Part print with two shaded views. Sizes in mm from the minimum x, y, z corner. Round coordinates to 2 decimals unless told otherwise and drop trailing zeros. Order: outer loops, then holes, each group sorted by start corner. A loop starts at its lowest first (then second) coordinate and runs counter-clockwise, first axis right, second up. Notation, with made-up numbers: (-26.5, 39) - (17.5, 39) arc R26 ccw to (17.5, 64) - close; hole circle Ø5 at (-14.75, -27). An arc over 180 degrees is marked (long way). Use one line per item in the form item = value.
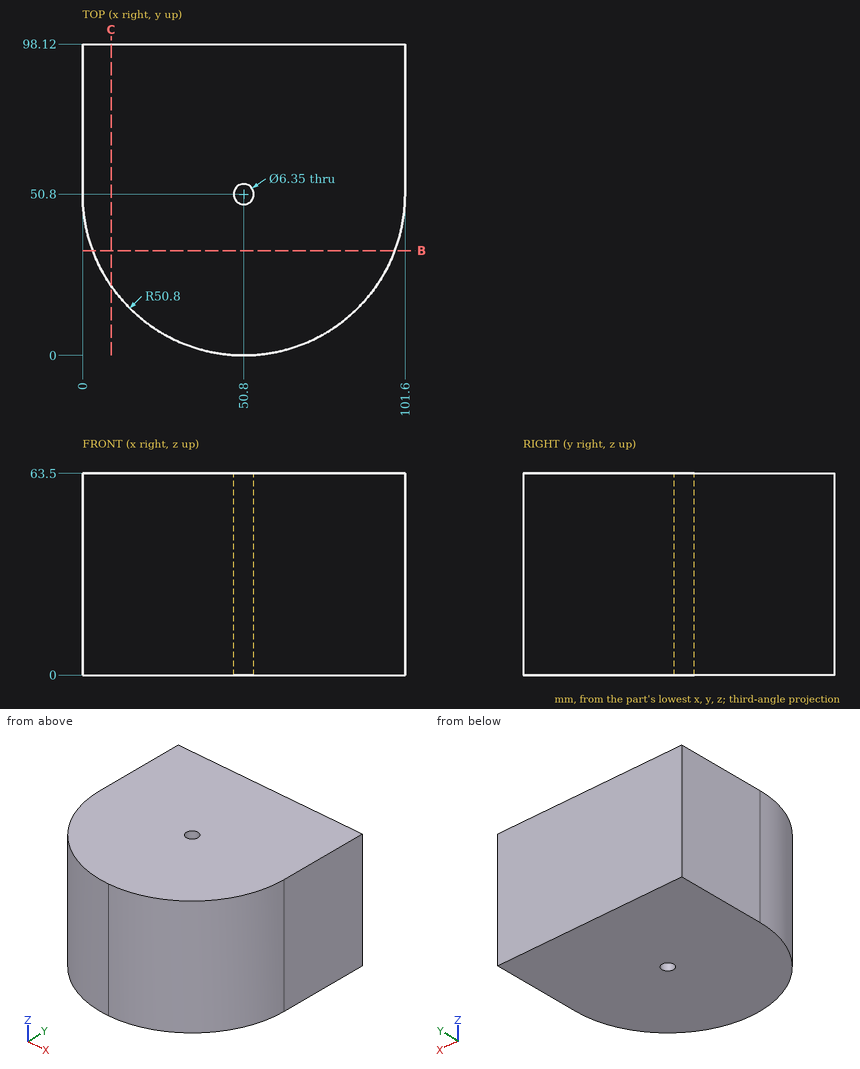
(1) Pin check, flat tips, straight feed: pin 1 (6 mm diameter, centred on x = 71, z = 56, fed in from -Y); pin 2 (4 mm diameter, centred on x = 50.8, y = 50.8, fed in from -Z); pin 3 (6 mm diameter, centred on x = 32, z = 36.5, fed in from -Y); pin 4 (6 mm diameter, centred on x = 33, z = 56.5, fed in from -Y). Stop position of each tip, or through.
Report:
pin_1 = 3
pin_2 = through
pin_3 = 2.52
pin_4 = 2.2
(2) Slice it at C-C on x = 9. Give the cut face in (y, z).
Report:
outline = (21.93, 0) - (98.12, 0) - (98.12, 63.5) - (21.93, 63.5) - close
(3) Probe probe 1 along Y at (x, z) = (50, 39); probe 2 along X at (y, z) = (49, 32.5) (1 decimal); probe 3 along X at (y, z) = (50, 42). List the from-to ranges inside material, lowest first. Write a range as [from, to].
Report:
probe_1 = [0.01, 47.73], [53.87, 98.12]
probe_2 = [0, 48.2], [53.4, 101.6]
probe_3 = [0.01, 47.73], [53.87, 101.59]
(4) Slice it at B-B on y = 33. Give the cut face in (x, z).
Report:
outline = (3.22, 0) - (98.38, 0) - (98.38, 63.5) - (3.22, 63.5) - close
